Could you check a few things on this model? Use its own coordinates, in mm. A direction names the side the tool comes from. Round coordinates to 2 decimals unless told otherwise and drop trailing zeros. Order: outer loops, then holes, each group sorted by start corner. A loop starts at its lowest first (then second) coordinate and runs counter-clockwise, first axis right, second up. Notation, with made-up numbers: (89, -6.75) -> (116, -6.75) arc R25 ccw to (116, 11.25) -> close; hole circle Ø4 at (84.5, -8). An arc over 180 degrees is marked (long way). One line per question, with ' | ' between items.
```python
from build123d import *

# Parameters (mm, degrees)
SKETCH_OPTIMIZATION_PARAMETERS_R = 1
BOSS_EXTRUDE1_DEPTH              = 12
SKETCH2_R                        = 3.3
CUT_EXTRUDE1_DEPTH               = 2.25
CUT_EXTRUDE1_DEPTH_BACK          = 2.25
HOLE_SKETCH_R                    = 1.288405797
SCREW_SHAFT_HOLES_DEPTH          = 5
SCREW_SHAFT_HOLES_DEPTH_BACK     = 10.763989156
SKETCH5_R                        = 2.38125
SCREW_COUNTERBORES_DEPTH         = 2.591836735


with BuildPart() as part:
    # Sketch-optimization parameters → Boss-Extrude1 (new body)
    with BuildSketch(Plane.XY):
        with BuildLine():
            Line((0, 0), (0, 20.103508611))
            Line((0, 20.103508611), (6.398918491, 20.103508611))
            ThreePointArc((6.398918491, 20.103508611), (9.29529716, 16.32184973), (4.889598418, 14.510835682))
            Line((4.889598418, 14.510835682), (4, 13.621237264))
            Line((4, 13.621237264), (4, 1.750446326))
            Line((4, 1.750446326), (4.889598418, 0.860847908))
            Line((4.889598418, 0.860847908), (7.778825692, 0.152757593))
            ThreePointArc((7.778825692, 0.152757593), (13.029319293, 2.417543543), (10.049883998, -2.463020336))
            Line((10.049883998, -2.463020336), (0, 0))
        make_face()
        with Locations((6.398918491, 17.103508611)):
            Circle(SKETCH_OPTIMIZATION_PARAMETERS_R, mode=Mode.SUBTRACT)
        with Locations((10.763989156, 0.450749356)):
            Circle(SKETCH_OPTIMIZATION_PARAMETERS_R, mode=Mode.SUBTRACT)
    extrude(amount=BOSS_EXTRUDE1_DEPTH)

    # Sketch2 → Cut-Extrude1 (cut, two sides)
    with BuildSketch(Plane.XY.offset(6)) as cut_extrude1_sk:
        with Locations((6.398918491, 17.103508611)):
            Circle(SKETCH2_R)
        with Locations((10.763989156, 0.450749356)):
            Circle(SKETCH2_R)
    extrude(amount=CUT_EXTRUDE1_DEPTH, mode=Mode.SUBTRACT)
    extrude(cut_extrude1_sk.sketch, amount=-CUT_EXTRUDE1_DEPTH_BACK, mode=Mode.SUBTRACT)

    # Hole sketch → Screw shaft holes (cut, two sides)
    with BuildSketch(Plane(origin=(4, 36.444645714, 0), x_dir=(0, 0, -1), z_dir=(-1, 0, 0))) as screw_shaft_holes_sk:
        with Locations((-9, 25.823408449)):
            Circle(HOLE_SKETCH_R)
        with Locations((-3, 25.823408449)):
            Circle(HOLE_SKETCH_R)
        with Locations((-6, 31.355067842)):
            Circle(HOLE_SKETCH_R)
    extrude(amount=SCREW_SHAFT_HOLES_DEPTH, mode=Mode.SUBTRACT)
    extrude(screw_shaft_holes_sk.sketch, amount=-SCREW_SHAFT_HOLES_DEPTH_BACK, mode=Mode.SUBTRACT)

    # Sketch5 → Screw counterbores (cut)
    with BuildSketch(Plane(origin=(4, 26.197134063, 0), x_dir=(0, 0, -1), z_dir=(-1, 0, 0))):
        with Locations((-6, 21.107556192)):
            Circle(SKETCH5_R)
        with Locations((-9, 15.575896799)):
            Circle(SKETCH5_R)
        with Locations((-3, 15.575896799)):
            Circle(SKETCH5_R)
    extrude(amount=SCREW_COUNTERBORES_DEPTH, mode=Mode.SUBTRACT)


solid = part.part
```
1. I'm going to push flat-ended pins straight in: pin 1 (1 mm diameter, centred on y = 1.5, z = 4, fed in from +X); pin 2 (6.5 mm diameter, centred on x = 10, y = 2, fed in from -Z); pin 3 (1.5 mm diameter, centred on x = 9, z = 6, fed in from +Y); pin 4 (1.4 mm diameter, centred on y = 11.5, z = 3, fed in from +X). Where does each tip first touch, or does it pass through?
From the geometry:
pin 1: stops at x = 13.7 | pin 2: stops at z = 0 | pin 3: stops at y = -1.69 | pin 4: stops at x = 1.41
2. I want a section at B-B on y = 16.5. List the corners of the cut face in (x, z) for me, and give its area (3 significant figures).
From the geometry:
outline: (0, 0) -> (5.6, 0) -> (5.6, 3.75) -> (3.15, 3.75) -> (3.15, 8.25) -> (5.6, 8.25) -> (5.6, 12) -> (0, 12) -> close; (7.2, 0) -> (9.34, 0) -> (9.34, 3.75) -> (7.2, 3.75) -> close; (7.2, 8.25) -> (9.34, 8.25) -> (9.34, 12) -> (7.2, 12) -> close | area: 72.3 mm²
3. If we mould it in two halves opening along Y, with no side actions, what happens to faces 4 (the face through (11, -1, 3.75)), 5 (the face through (3.11, 17.35, 6.03))? For each: pulls with the +Y half, pulls with the -Y half, needs draft (parallel to the pull), parting line crosses it, or undercut.
From the geometry:
face 4: needs draft | face 5: undercut
4. I want a section at C-C on x = 10.5. List the corners of the cut face in (y, z) for me, and give its area (3 significant figures).
From the geometry:
outline: (-2.54, 0) -> (-0.51, 0) -> (-0.51, 3.75) -> (-2.54, 3.75) -> close; (-2.54, 8.25) -> (-0.51, 8.25) -> (-0.51, 12) -> (-2.54, 12) -> close; (1.42, 0) -> (3.44, 0) -> (3.44, 3.75) -> (1.42, 3.75) -> close; (1.42, 8.25) -> (3.44, 8.25) -> (3.44, 12) -> (1.42, 12) -> close | area: 30.4 mm²
5. On a 3-axis mill with a long thin cutter (end or side, diameter ignored), from which of +Z, -Z, +X, -X, +Y, -Y can I reach the whole of each face in a straight line? I mean faces 1 (the face through (2, 9, 0)), 2 (the face through (4.44, 1.31, 5.92)), 3 (the face through (1.408, 12, 2)). Say none if no direction works.
From the geometry:
face 1: -Z, +X, -X, +Y, -Y | face 2: +Z, -Z | face 3: +X
6. I want a section at D-D on z = 6. List the corners of the cut face in (x, y) for me, and give its area (3 significant figures).
From the geometry:
outline: (0, 0) -> (8.71, -2.14) arc R3.3 cw to (7.47, 0.23) -> (4.89, 0.86) -> (4, 1.75) -> (4, 2.71) -> (1.41, 2.71) -> (1.41, 3.8) -> (0, 3.8) -> close; (0, 6.38) -> (1.41, 6.38) -> (1.41, 7.47) -> (4, 7.47) -> (4, 13.62) -> (4.67, 14.29) arc R3.3 cw to (5.02, 20.1) -> (0, 20.1) -> close | area: 72.5 mm²
7. I need wall thicknesses on probe 1 along Y at (x, z) = (2.25, 9); probe 2 along Z at (x, y) = (1.5, 12); probe 3 along Y at (x, z) = (7, 3.5). Which ranges of each line are inside material? Lowest first, please.
From the geometry:
probe 1: y = -0.55 to 8.24, 13 to 20.1 | probe 2: z = 0 to 1.06, 4.94 to 7.06, 10.94 to 12 | probe 3: y = -1.72 to 0.34, 14.16 to 16.3, 17.9 to 20.04
8. I want a section at A-A on z = 10. List the corners of the cut face in (x, y) for me, and give its area (3 significant figures).
From the geometry:
outline: (0, 0) -> (10.05, -2.46) arc R3 ccw (long way) to (7.78, 0.15) -> (4.89, 0.86) -> (4, 1.75) -> (4, 8.46) -> (1.41, 8.46) -> (1.41, 9.81) -> (0, 9.81) -> close; (0, 11.43) -> (1.41, 11.43) -> (1.41, 12.78) -> (4, 12.78) -> (4, 13.62) -> (4.89, 14.51) arc R3 ccw (long way) to (6.4, 20.1) -> (0, 20.1) -> close; hole circle Ø2 at (6.4, 17.1); hole circle Ø2 at (10.76, 0.45) | area: 128 mm²
